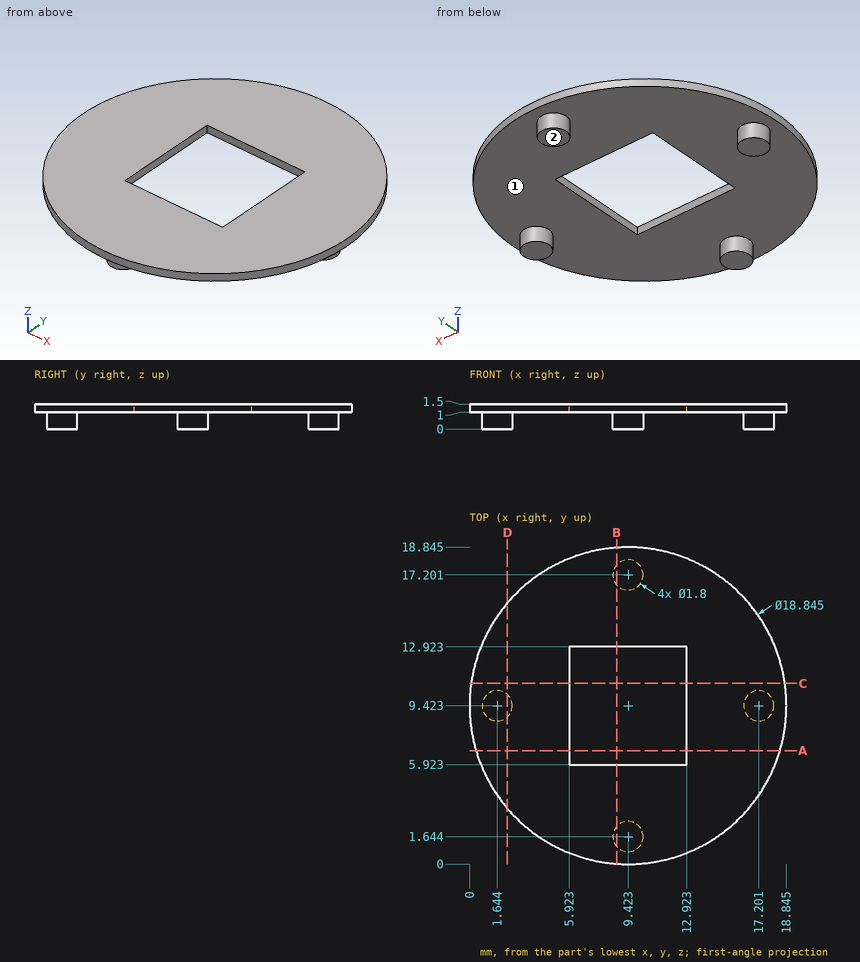
Check sheet for the drawn part. Datum: minimum x, y, z corner. Units: mm. A direction names the side the tool comes from. Give positions to 0.01 mm unless a question says otherwise; leave off trailing zeros. Order: outer loops, then holes, each group sorted by start corner. A loop starts at its lowest first (then second) coordinate and runs counter-clockwise, first axis right, second up. Notation, with made-up numbers: (89, 79) -> (105, 79) arc R18 cw to (105, 84) -> close; hole circle Ø4 at (67, 19). An arc over 180 degrees is marked (long way). Use a Markdown table: item, result.
1) Section check C-C, the plane y = 10.75. Record the boundary of the cut face in (x, z).
Results:
| item | result |
|---|---|
| outline | (0.09, 1) -> (5.92, 1) -> (5.92, 1.5) -> (0.09, 1.5) -> close; (12.92, 1) -> (18.75, 1) -> (18.75, 1.5) -> (12.92, 1.5) -> close |
2) Tool access check on the marked faces 1 and 2. Record the directions out of +Z, -Z, +X, -X, +Y, -Y that give a thin tool (end or side, any length) a straight path to the whole face; none if there is none.
Results:
| item | result |
|---|---|
| face 1 | -Z |
| face 2 | -Z, +X, -X, +Y, -Y |
3) Section check A-A, the plane y = 6.75. Record the boundary of the cut face in (x, z).
Results:
| item | result |
|---|---|
| outline | (0.39, 1) -> (5.92, 1) -> (5.92, 1.5) -> (0.39, 1.5) -> close; (12.92, 1) -> (18.46, 1) -> (18.46, 1.5) -> (12.92, 1.5) -> close |
4) Section check D-D, the plane x = 2.25. Record the boundary of the cut face in (y, z).
Results:
| item | result |
|---|---|
| outline | (3.31, 1) -> (8.76, 1) -> (8.76, 0) -> (10.09, 0) -> (10.09, 1) -> (15.53, 1) -> (15.53, 1.5) -> (3.31, 1.5) -> close |
5) Depth check by flat-ended pin: pin 1 Ø0.6 at (x, z) = (10, 1.5) entering from +Y; pin 2 Ø5 at (x, y) = (2.5, 4) entering from -Z. Enter the tip coordinate at first touch or a pass-through.
Results:
| item | result |
|---|---|
| pin 1 | y = 18.84 |
| pin 2 | z = 1 |
6) Section check B-B, the plane x = 8.75. Record the boundary of the cut face in (y, z).
Results:
| item | result |
|---|---|
| outline | (0.02, 1) -> (1.05, 1) -> (1.05, 0) -> (2.24, 0) -> (2.24, 1) -> (5.92, 1) -> (5.92, 1.5) -> (0.02, 1.5) -> close; (12.92, 1) -> (16.6, 1) -> (16.6, 0) -> (17.8, 0) -> (17.8, 1) -> (18.82, 1) -> (18.82, 1.5) -> (12.92, 1.5) -> close |
7) Material ranges on probe 1 along Z at (x, y) = (3.75, 3.5); probe 2 along X at (y, z) = (12.5, 1.2); probe 3 along X at (y, z) = (17.25, 0.25), recorded low to high.
Results:
| item | result |
|---|---|
| probe 1 | 1 to 1.5 |
| probe 2 | 0.52 to 5.92, 12.92 to 18.33 |
| probe 3 | 8.52 to 10.32 |
